from build123d import *

# Parameters (mm, degrees)
F0_R     = 298.45
F0_R_2   = 14.351
F0_R_3   = 205.232
F1_DEPTH = 36.576
F2_R     = 234.95
F2_R_2   = 205.232
F3_DEPTH = 1.5875
F4_R     = 228.6
F4_R_2   = 205.232
F5_DEPTH = 26.924
F6_R     = 2.54


with BuildPart() as f1:
    # F0 (on Front) → F1 (new body)
    with BuildSketch(Plane.XZ):
        Circle(F0_R)
        with Locations((-149.934517, -224.392862)):
            Circle(F0_R_2, mode=Mode.SUBTRACT)
        with Locations((-224.392862, -149.934517)):
            Circle(F0_R_2, mode=Mode.SUBTRACT)
        with Locations((-52.650001, -264.689428)):
            Circle(F0_R_2, mode=Mode.SUBTRACT)
        with Locations((-264.689428, -52.650001)):
            Circle(F0_R_2, mode=Mode.SUBTRACT)
        with Locations((52.650001, -264.689428)):
            Circle(F0_R_2, mode=Mode.SUBTRACT)
        with Locations((149.934517, -224.392862)):
            Circle(F0_R_2, mode=Mode.SUBTRACT)
        with Locations((224.392862, -149.934517)):
            Circle(F0_R_2, mode=Mode.SUBTRACT)
        with Locations((264.689428, -52.650001)):
            Circle(F0_R_2, mode=Mode.SUBTRACT)
        with Locations((-264.689428, 52.650001)):
            Circle(F0_R_2, mode=Mode.SUBTRACT)
        with Locations((-224.392862, 149.934517)):
            Circle(F0_R_2, mode=Mode.SUBTRACT)
        with Locations((-149.934517, 224.392862)):
            Circle(F0_R_2, mode=Mode.SUBTRACT)
        with Locations((-52.650001, 264.689428)):
            Circle(F0_R_2, mode=Mode.SUBTRACT)
        Circle(F0_R_3, mode=Mode.SUBTRACT)
        with Locations((264.689428, 52.650001)):
            Circle(F0_R_2, mode=Mode.SUBTRACT)
        with Locations((52.650001, 264.689428)):
            Circle(F0_R_2, mode=Mode.SUBTRACT)
        with Locations((224.392862, 149.934517)):
            Circle(F0_R_2, mode=Mode.SUBTRACT)
        with Locations((149.934517, 224.392862)):
            Circle(F0_R_2, mode=Mode.SUBTRACT)
    extrude(amount=F1_DEPTH)

    # F2 (on face) → F3 (join)
    with BuildSketch(Plane.XZ.offset(36.576)):
        Circle(F2_R)
        Circle(F2_R_2, mode=Mode.SUBTRACT)
    extrude(amount=F3_DEPTH)

    # F4 (on face) → F5 (join)
    with BuildSketch(Plane(origin=(0, 0, 0), x_dir=(-1, 0, 0), z_dir=(0, 1, 0))):
        Circle(F4_R)
        Circle(F4_R_2, mode=Mode.SUBTRACT)
    extrude(amount=F5_DEPTH)

    # F6
    f6_edges = [f1.edges().sort_by_distance(p)[0] for p in [
        (-298.45, 0, 0),
        (205.232, 26.924, 0),
        (-298.45, -36.576, 0),
        (-205.232, -38.1635, 0),
    ]]
    fillet(f6_edges, radius=F6_R)


solid = f1.part
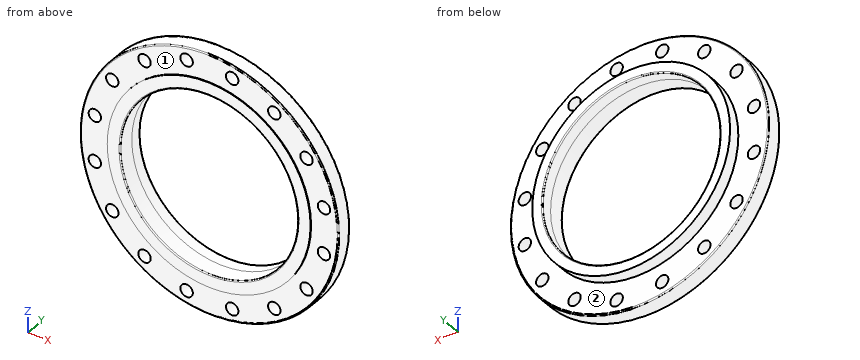
The model under review builds one solid part; all positions refer to its coordinate system, in mm. Face numbers are marked on the shaded views. A direction names the side the tool comes from. Coordinates: 2 decimals unless noted, no trailing zeros. Loops run counter-clockwise (first coordinate to the right, second up) from the corner with the lowest first, then second, coordinate; pieces in that order, holes last. Notation, with made-up numbers: (-19.75, -15.75) -> (9.25, -15.75) arc R11 cw to (9.25, -8.75) -> close; hole circle Ø11 at (15.25, 68). An arc over 180 degrees is marked (long way). Use a Markdown table: item, result. Add a question column.
1. Add section C-C on y = 9. Write out the cut boundary in (x, z), plus the area to 3 significant figures.
2. Clearance check with flat-ended pins moving along their axes: pin 1 Ø1 at (x, y) = (132, -18.5) entering from +Z; pin 2 Ø1.5 at (y, z) = (-8.5, 118.5) entering from -X; pin 3 Ø6 at (y, z) = (-28.5, 75) entering from +X; pin 4 Ø17 at (x, z) = (-224.39, 149.93) entering from -Y. State where each tip first meets the part, or that it passes through.
3. Add section A-A on x = 0. Write out the cut boundary in (y, z), plus the area to 3 significant figures.
4. Add section D-D on y = -24. Give the number of separate pieces and of enclosed holes in the cut face, plus the area to 3 significant figures.
5. To check wall thickness, follow line 1 (Z direction, x = 0, y = -11); line 2 (X direction, y = -0.5, z = -212); line 3 (X direction, y = -22, z = -142.5). State the ranges of each line that lie inside material, in increasing order.
6. Machinability: for the marked faces 1 and 2, which of the approach directions +Z, -Z, +X, -X, +Y, -Y give a long, thin tool a straight path to every point of the face, cutting with its end or side? Answer none if there is none.
7. Add section B-B on z = 0. Write out the cut boundary in (x, y), plus the area to 3 significant figures.
Returned:
| question | item | result |
|---|---|---|
| 1 | outline | circle Ø457.2 at (0, 0); hole circle Ø410.46 at (0, 0) |
| 1 | area | 31,800 mm² |
| 2 | pin 1 | stops at z = 267.92 |
| 2 | pin 2 | stops at x = -274.24 |
| 2 | pin 3 | stops at x = 289.63 |
| 2 | pin 4 | passes through |
| 3 | outline | (-38.16, -234.95) -> (-36.58, -234.95) -> (-36.58, -295.91) arc R2.54 ccw to (-34.04, -298.45) -> (-2.54, -298.45) arc R2.54 ccw to (0, -295.91) -> (0, -228.6) -> (26.92, -228.6) -> (26.92, -207.77) arc R2.54 ccw to (24.38, -205.23) -> (-35.62, -205.23) arc R2.54 ccw to (-38.16, -207.77) -> close; (-38.16, 207.77) arc R2.54 ccw to (-35.62, 205.23) -> (24.38, 205.23) arc R2.54 ccw to (26.92, 207.77) -> (26.92, 228.6) -> (0, 228.6) -> (0, 295.91) arc R2.54 ccw to (-2.54, 298.45) -> (-34.04, 298.45) arc R2.54 ccw to (-36.58, 295.91) -> (-36.58, 234.95) -> (-38.16, 234.95) -> close |
| 3 | area | 8,160 mm² |
| 4 | separate pieces | 1 |
| 4 | enclosed holes | 17 |
| 4 | area | 137,000 mm² |
| 5 | line 1 | z = -298.45 to -205.23, 205.23 to 298.45 |
| 5 | line 2 | x = -208.61 to -157.17, -142.7 to 142.7, 157.17 to 208.61 |
| 5 | line 3 | x = -262.23 to -236.67, -212.12 to -147.7, 147.7 to 212.12, 236.67 to 262.23 |
| 6 | face 1 | -Y |
| 6 | face 2 | +Y |
| 7 | outline | (-298.45, -34.04) arc R2.54 ccw to (-295.91, -36.58) -> (-234.95, -36.58) -> (-234.95, -38.16) -> (-207.77, -38.16) arc R2.54 ccw to (-205.23, -35.62) -> (-205.23, 24.38) arc R2.54 ccw to (-207.77, 26.92) -> (-228.6, 26.92) -> (-228.6, 0) -> (-295.91, 0) arc R2.54 ccw to (-298.45, -2.54) -> close; (205.23, -35.62) arc R2.54 ccw to (207.77, -38.16) -> (234.95, -38.16) -> (234.95, -36.58) -> (295.91, -36.58) arc R2.54 ccw to (298.45, -34.04) -> (298.45, -2.54) arc R2.54 ccw to (295.91, 0) -> (228.6, 0) -> (228.6, 26.92) -> (207.77, 26.92) arc R2.54 ccw to (205.23, 24.38) -> close |
| 7 | area | 8,160 mm² |
